from build123d import *

# Parameters (mm, degrees)
SKETCH1_R                = 203.2
BOSS_EXTRUDE1_DEPTH      = 101.6
SKETCH3_R                = 76.2
BOSS_EXTRUDE2_DEPTH      = 101.6
BOSS_EXTRUDE2_DEPTH_BACK = 203.2
SKETCH4_R                = 19.05
CUT_EXTRUDE2_DEPTH       = 305.8
SKETCH5_R                = 38.1
CUT_EXTRUDE3_DEPTH       = 101.6
CIRPATTERN1_COUNT        = 8
FILLET1_R                = 12.7
FILLET2_R                = 12.7
CUT_EXTRUDE4_REACH       = 408.4
SKETCH6_R                = 6.35
CUT_EXTRUDE5_REACH       = 408.4
SKETCH7_R                = 6.35
SKETCH8_R                = 25.4
CUT_EXTRUDE6_DEPTH       = 12.7
SKETCH9_R                = 25.4
CUT_EXTRUDE7_DEPTH       = 12.7


with BuildPart() as part:
    # Sketch1 → Boss-Extrude1 (new body)
    with BuildSketch(Plane.XY):
        Circle(SKETCH1_R)
    extrude(amount=BOSS_EXTRUDE1_DEPTH)

    # Sketch3 → Boss-Extrude2 (add, two sides)
    with BuildSketch(Plane.XY.offset(101.6)) as boss_extrude2_sk:
        Circle(SKETCH3_R)
    extrude(amount=BOSS_EXTRUDE2_DEPTH)
    extrude(boss_extrude2_sk.sketch, amount=-BOSS_EXTRUDE2_DEPTH_BACK)

    # Sketch4 → Cut-Extrude2 (cut, through all)
    with BuildSketch(Plane.XY.offset(203.2)):
        Circle(SKETCH4_R)
    extrude(amount=-CUT_EXTRUDE2_DEPTH, mode=Mode.SUBTRACT)

    # Sketch5 → Cut-Extrude3 (cut)
    with BuildSketch(Plane.XY.offset(101.6)):
        with Locations((0, 139.7)):
            Circle(SKETCH5_R)
    cut_extrude3 = extrude(amount=-CUT_EXTRUDE3_DEPTH, mode=Mode.SUBTRACT)

    # CirPattern1: Cut-Extrude3 ×8 about axis
    cirpattern1_axis = Axis((0, 0, 0), (0, 0, 1))
    for i in range(1, CIRPATTERN1_COUNT):
        add(cut_extrude3.rotate(cirpattern1_axis, i * 360 / CIRPATTERN1_COUNT), mode=Mode.SUBTRACT)

    # Fillet1
    fillet1_edges = [part.edges().sort_by_distance(p)[0] for p in [
        (-76.2, 0, 101.6),
    ]]
    fillet(fillet1_edges, radius=FILLET1_R)

    # Fillet2
    fillet2_edges = [part.edges().sort_by_distance(p)[0] for p in [
        (-76.2, 0, 0),
        (-76.2, 0, -101.6),
        (-76.2, 0, 203.2),
    ]]
    fillet(fillet2_edges, radius=FILLET2_R)

    # Sketch6 → Cut-Extrude4 (cut, up to next)
    with BuildSketch(Plane(origin=(0, 203.2, 0), x_dir=(-1, 0, 0), z_dir=(0, 1, 0)), mode=Mode.PRIVATE) as cut_extrude4_sk1:
        with Locations((0, 50.8)):
            Circle(SKETCH6_R)
    cut_extrude4_tool1 = extrude(cut_extrude4_sk1.sketch, amount=-CUT_EXTRUDE4_REACH, mode=Mode.PRIVATE) & part.part
    add(cut_extrude4_tool1.solids().sort_by_distance((0, 203.2, 50.8))[0], mode=Mode.SUBTRACT)

    # Sketch7 → Cut-Extrude5 (cut, up to next)
    with BuildSketch(Plane.XZ.offset(203.2), mode=Mode.PRIVATE) as cut_extrude5_sk1:
        with Locations((0, 50.8)):
            Circle(SKETCH7_R)
    cut_extrude5_tool1 = extrude(cut_extrude5_sk1.sketch, amount=-CUT_EXTRUDE5_REACH, mode=Mode.PRIVATE) & part.part
    add(cut_extrude5_tool1.solids().sort_by_distance((0, -203.2, 50.8))[0], mode=Mode.SUBTRACT)

    # Sketch8 → Cut-Extrude6 (cut)
    with BuildSketch(Plane.XY.offset(203.2)):
        Circle(SKETCH8_R)
    extrude(amount=-CUT_EXTRUDE6_DEPTH, mode=Mode.SUBTRACT)

    # Sketch9 → Cut-Extrude7 (cut)
    with BuildSketch(Plane(origin=(0, 0, -101.6), x_dir=(-1, 0, 0), z_dir=(0, 0, -1))):
        Circle(SKETCH9_R)
    extrude(amount=-CUT_EXTRUDE7_DEPTH, mode=Mode.SUBTRACT)


solid = part.part
The listing builds one solid part. Answer for the finished solid, in the listing's coordinates (mm). A direction names the side the tool comes from. Coordinates: 2 decimals unless noted, no trailing zeros. Write each loop counter-clockwise with the first axis right and the second up, starting at its lowest first coordinate (ties: lowest second). Pieces come first, ordered by that corner, then holes. Notation, with made-up numbers: M 8.25,-23.5 L 22.25,-23.5 A15 ccw 22.25,-9.5 Z; hole C -25,89.5 d8. An arc over 180 degrees is marked long. Put each result on its own line as item: value. Start each with the question number.
1. For a pull along Y with two mould halves and no side action, classify faces 1 (the flat face through (-93, 3, 101.6)), 2 (the cylindrical face through (177.476, 4.96, 51.511)), 3 (the cylindrical face through (-15.12, -11.59, 52.76)), 4 (the cylindrical face through (-60.47, -46.367, -50.267)) as pulls with the +Y half, pulls with the -Y half, needs draft (parallel to the pull), parting line crosses it, or undercut.
2. A cutting plane is placed at B-B on z = 50.8. Write down the section's boundary in (x, y), then the cut area to 3 significant figures.
3. A cutting plane is placed at D-D on z = 168. Write down the section's boundary in (x, y).
4. Consider line 1 (Z direction, x = 0, y = 198.25); line 2 (Y direction, x = -16, z = 31.5); line 3 (Z direction, x = 172.5, y = -52). Determine where each line is inside the solid, lowest interval first. Write a range as from..to.
5. Flat-ended cylindrical pins translate along their axes: P1, Ø8, axis at x = -105, z = 91.5, coming from the +Y side; P2, Ø5, axis at y = 98.5, z = 8.5, coming from the +X side; P3, Ø12, axis at y = -54, z = -7.5, coming from the -X side; P4, Ø14.5, axis at x = 0, z = 50.8, coming from the -Y side. Find the tip coordinate at first contact, or state that the pin passes through.
6. A cutting plane is placed at A-A on y = 0. Count the separate pieces of the cut face and the enclosed holes in it, then the cut area to 3 significant figures.
7. Which of the six approach directions +Z, -Z, +X, -X, +Y, -Y give full straight-line access (tool end or side, diameter ignored) to faces 5 (the flat face through (27, 1, -101.6)), 6 (the cylindrical face through (-0.8, -190.4, 57.1)), 7 (the cylindrical face through (0.8, 190.4, 57.1)), 8 (the flat face through (-4, 19, -88.9)), 9 (the flat face through (4, 19, 190.5))?
Resolved:
1. face 1: needs draft
1. face 2: undercut
1. face 3: undercut
1. face 4: parting line crosses it
2. outline: M -6.35,-203.1 L -6.35,-177.27 A38.1 cw long 6.35,-177.27 L 6.35,-203.1 A203.2 ccw 6.35,203.1 L 6.35,177.27 A38.1 cw long -6.35,177.27 L -6.35,203.1 A203.2 ccw Z; hole C -139.7,0 d76.2; hole C -98.78,-98.78 d76.2; hole C -98.78,98.78 d76.2; hole C 0,0 d38.1; hole C 98.78,-98.78 d76.2; hole C 98.78,98.78 d76.2; hole C 139.7,0 d76.2
2. area: 91,400 mm2
3. outline: C 0,0 d152.4; hole C 0,0 d38.1
4. line 1: z = 0..44.45, 57.15..101.6
4. line 2: y = -202.57..-174.28, -105.12..-10.34, 10.34..105.12, 174.28..202.57
4. line 3: z = 0..101.6
5. P1: stops at y = 176.32
5. P2: stops at x = 179.09
5. P3: stops at x = -63.81
5. P4: stops at y = -203.2
6. separate pieces: 4
6. enclosed holes: 0
6. area: 44,800 mm2
7. face 5: -Z, +X, -X, +Y, -Y
7. face 6: -Y
7. face 7: +Y
7. face 8: -Z
7. face 9: +Z
